Check sheet for the modelled part. Datum: model origin and axes. Units: mm. Face numbers are marked on the shaded views. A direction names the side the tool comes from. Round coordinates to 2 decimals unless told otherwise and drop trailing zeros. Order: outer loops, then holes, each group sorted by start corner. A loop starts at its lowest first (then second) coordinate and runs counter-clockwise, first axis right, second up.
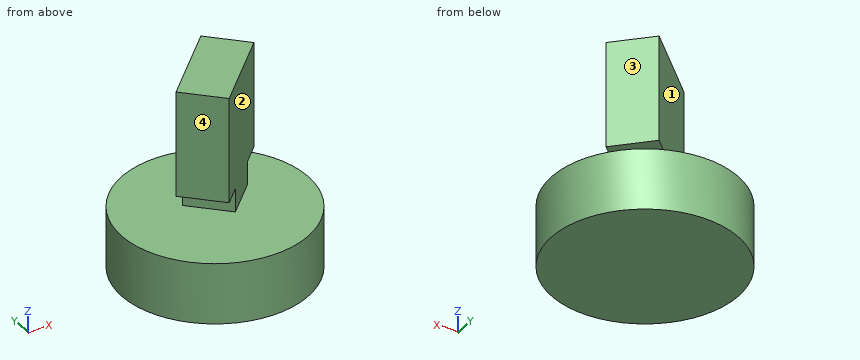
```python
from build123d import *

# Parameters (mm, degrees)
SKETCH_1_R      = 40
EXTRUDE_1_DEPTH = 26
SKETCH_2_R      = 1.5
EXTRUDE_2_DEPTH = 5
EXTRUDE_3_DEPTH = 10
EXTRUDE_4_DEPTH = 45


with BuildPart() as part:
    # 草图1 → 凸台-拉伸1 (new body)
    with BuildSketch(Plane.XY):
        with Locations(Location((0, 0, 0), (0, 0, 180))):
            Circle(SKETCH_1_R)
    extrude(amount=EXTRUDE_1_DEPTH)

    # 草图2 → 凸台-拉伸2 (add)
    with BuildSketch(Plane.XY.offset(26)):
        Circle(SKETCH_2_R)
    extrude(amount=EXTRUDE_2_DEPTH)

    # 草图3 → 凸台-拉伸3 (add)
    with BuildSketch(Plane.XY.offset(31)):
        Polygon((0, 14.14), (14.14, 0), (0, -14.14), (-14.14, 0), align=None)
    extrude(amount=EXTRUDE_3_DEPTH)

    # 草图5 → 凸台-拉伸4 (add)
    with BuildSketch(Plane.XY.offset(41)):
        Polygon((0, -14.14), (-14.14, 0), (-21.213203436, -7.073203436), (-7.073203436, -21.213203436), align=None)
        Polygon((7.073203436, 21.213203436), (0, 14.14), (14.14, 0), (21.213203436, 7.073203436), align=None)
        Polygon((14.14, 0), (0, 14.14), (-14.14, 0), (0, -14.14), align=None)
    extrude(amount=EXTRUDE_4_DEPTH)


solid = part.part
```
Item 1: Go/stop test with flat-tipped pins: P1, Ø12, axis at x = -21.5, z = 62, coming from the -Y side; P2, Ø10, axis at x = 15, z = 15.5, coming from the +Y side; P3, Ø3, axis at y = 9, z = 64.5, coming from the -X side. Record where each tip stops, or that it passes through.
Answer:
P1: stops at y = -12.79
P2: stops at y = 38.73
P3: stops at x = -6.64
Item 2: Sectioned sample at B-B (z = 73.5). Record the cut outline in (x, y), and give its area (3 significant figures).
Answer:
outline: (-21.21, -7.07) - (-7.07, -21.21) - (21.21, 7.07) - (7.07, 21.21) - close
area: 800 mm2
Item 3: Sectioned sample at A-A (x = -9). Record the cut outline in (y, z).
Answer:
outline: (-38.97, 0) - (38.97, 0) - (38.97, 26) - (-38.97, 26) - close; (-19.29, 41) - (-5.14, 41) - (-5.14, 31) - (5.14, 31) - (5.14, 86) - (-19.29, 86) - close
Item 4: Sectioned sample at C-C (y = -28). Record the cut outline in (x, z).
Answer:
outline: (-28.57, 0) - (28.57, 0) - (28.57, 26) - (-28.57, 26) - close
Item 5: Scan lines: line 1 along Z through (x, y) = (4, -7); line 2 along Z through (x, y) = (-9, -15); line 3 along Z through (x, y) = (-8, 33). Record each from-to range of solid material in increasing order.
Answer:
line 1: z = 0 to 26, 31 to 86
line 2: z = 0 to 26, 41 to 86
line 3: z = 0 to 26
Item 6: Access from +Z, -Z, +X, -X, +Y, -Y to the whole of each face (thin tool, end or side, straight path). Record for the marked faces 1, 2, 3 and 4.
Answer:
face 1: +Z, -X, +Y
face 2: +Z, +X, -Y
face 3: +Z, +X, +Y
face 4: +Z, -X, -Y
